Here's how the part is built. I have some questions about the finished solid (model axes, mm). A direction names the side the tool comes from. Coordinates: 2 decimals unless noted, no trailing zeros. Write each loop counter-clockwise with the first axis right and the second up, starting at its lowest first coordinate (ties: lowest second). Pieces come first, ordered by that corner, then holes. Notation, with made-up numbers: (27.5, 65) - (56.5, 65) arc R27 ccw to (56.5, 81) - close; hole circle Ø2 at (63, 72.25). An arc over 180 degrees is marked (long way). Answer in a Markdown table with one row per item. Add a question column.
Item 1: If I drill on probe 1 along Z at (x, y) = (-100, -157.5); probe 2 along Y at (x, z) = (-41.5, 47.5); probe 3 along Z at (x, y) = (31, -197.5), over which ranges is the centre line in solid material (lowest first)? Write a range as from..to.
Item 2: I'm going to push flat-ended pins straight in: pin 1 (20 mm diameter, centred on x = -41, z = 20.5, fed in from +Y); pin 2 (24.5 mm diameter, centred on x = -78, y = -129, fed in from -Z); pin 3 (12 mm diameter, centred on x = -72.5, z = -46.5, fed in from +Y). Where does each tip first touch, or does it pass through?
Item 3: We'd pull the mould along Z, two halves only. Please class faces 4 (the face through (-52, -140, -60)), 5 (the face through (-80, -141, 50)), 6 (the face through (-59.985, -83.479, 1.319)), 7 (the face through (-63, 3, -55)): +Z half, -Z half, draft (parallel to the pull), parting line (faces both ways), or undercut.
Item 4: Which directions (+Z, -Z, +X, -X, +Y, -Y) give clear straight access to the entire face, cutting with the end or side of a thin tool? Please do faces 1 (the face through (-61, -69, 0)), 2 (the face through (-83.3, -124.5, 55.1)), 3 (the face through (-68, -6, 50)).
Item 5: Imagine slicing it at C-C (z = 56). State how many separate pieces and enclosed holes the cut face has, plus the area to 3 significant figures.
Item 6: Imagine slicing it at A-A (x = -77). Please give me the cut outline in (y, z), plus the area to 3 significant figures.
Item 7: Imagine slicing it at B-B (y = -199.5). Please give me the cut outline in (x, z), plus the area to 3 significant figures.
from build123d import *

# Parameters (mm, degrees)
BOSS_EXTRUDE1_DEPTH      = 110
REVOLVE4_ANGLE           = 180
SKETCH5_R                = 2.5
BOSS_EXTRUDE2_DEPTH      = 120
CUT_EXTRUDE2_REACH       = 151.317
CUT_EXTRUDE2_END_RADIUS  = 50
REVOLVE5_ANGLE           = 180
CUT_EXTRUDE4_DEPTH       = 15
CUT_EXTRUDE5_DEPTH       = 85
CUT_EXTRUDE5_DEPTH_BACK  = 75
SKETCH7_5_W              = 21.213203436
SKETCH7_5_H              = 100
REVOLVE6_ANGLE           = 180
BOSS_EXTRUDE3_DEPTH      = 3
BOSS_EXTRUDE3_DEPTH_BACK = 10
SKETCH9_R                = 50
BOSS_EXTRUDE4_START      = -110
SKETCH9_3_R              = 50
BOSS_EXTRUDE4_DEPTH      = 13
BOSS_EXTRUDE5_DEPTH      = 120
CUT_EXTRUDE6_START       = -110
CUT_EXTRUDE6_DEPTH       = 20
CUT_EXTRUDE7_DEPTH       = 50
SKETCH9_5_R              = 7.5
BOSS_EXTRUDE6_DEPTH      = 10
BOSS_EXTRUDE7_START      = -110
SKETCH9_6_R              = 7.5
BOSS_EXTRUDE7_DEPTH      = 10
SKETCH12_R               = 12.571901436
CUT_EXTRUDE8_DEPTH       = 281.297435946
BOSS_EXTRUDE9_START      = 15
BOSS_EXTRUDE9_DEPTH      = 15


# Read off the part's stored shape, not the designer's step: Cut-Extrude6
with BuildPart() as part:
    # Sketch1 → Boss-Extrude1 (new body)
    with BuildSketch(Plane(origin=(0, 0, 0), x_dir=(1, 0, 0), z_dir=(0, 1, 0))):
        with BuildLine():
            Line((0, 60), (0, 50))
            ThreePointArc((0, 50), (-50, 0), (0, -50))
            Line((0, -50), (0, -60))
            ThreePointArc((0, -60), (-60, 0), (0, 60))
        make_face()
    extrude(amount=-BOSS_EXTRUDE1_DEPTH)

    # Sketch2 → Revolve4 (revolve)
    with BuildSketch(Plane(origin=(0, 0, 0), x_dir=(0, 0, -1), z_dir=(1, 0, 0))):
        with BuildLine():
            ThreePointArc((-7.741180955, 11.323216436), (-7.20664666, 11.680380834), (-7, 12.289142263))
            Line((-7, 12.289142263), (-7, 13.397459622))
            Line((-7, 13.397459622), (-5, 13.397459622))
            Line((-5, 13.397459622), (-5, 12.057713659))
            Line((-5, 12.057713659), (-5, 10.754488287))
            ThreePointArc((-5, 10.754488287), (-5.20664666, 10.145726858), (-5.741180955, 9.78856246))
            Line((-5.741180955, 9.78856246), (-49.872833452, -2.036478187))
            ThreePointArc((-49.872833452, -2.036478187), (-50.001126305, -2.061997222), (-50.131652498, -2.070552361))
            Line((-50.131652498, -2.070552361), (-60, -2.070552361))
            Line((-60, -2.070552361), (-60, 0))
            Line((-60, 0), (-50.131652498, 0))
            ThreePointArc((-50.131652498, 0), (-50.001126305, 0.008555139), (-49.872833452, 0.034074174))
            Line((-49.872833452, 0.034074174), (-7.741180955, 11.323216436))
        make_face()
    revolve(axis=Axis((0, 9.451262914, 0), (0, -1, 0)), revolution_arc=REVOLVE4_ANGLE)

    # Sketch5 → Boss-Extrude2 (add)
    with BuildSketch(Plane.XY.offset(60)):
        with BuildLine():
            Line((-60, -25), (0, -25))
            Line((0, -25), (0, -15))
            Line((0, -15), (0, 0))
            Line((0, 0), (-60, 0))
            Line((-60, 0), (-65.17766953, 5.17766953))
            ThreePointArc((-65.17766953, 5.17766953), (-68.713203436, 6.642135624), (-72.248737342, 5.17766953))
            Line((-72.248737342, 5.17766953), (-76.213203436, 1.213203436))
            Line((-76.213203436, 1.213203436), (-81.213203436, -3.786796564))
            Line((-81.213203436, -3.786796564), (-60, -25))
        make_face()
        with Locations((-68.713203436, 1.642135624)):
            Circle(SKETCH5_R, mode=Mode.SUBTRACT)
    extrude(amount=-BOSS_EXTRUDE2_DEPTH)

    # Cut-Extrude2: up to this cylinder (the profile starts inside it)
    cut_extrude2_end = Plane(origin=(0, -12.579447, 0), z_dir=(0, 1, 0)) * Cylinder(CUT_EXTRUDE2_END_RADIUS, 403.634, mode=Mode.PRIVATE)
    # Sketch6 → Cut-Extrude2 (cut, up to the surface)
    with BuildSketch(Plane(origin=(0, 0, 0), x_dir=(0, 0, -1), z_dir=(1, 0, 0)), mode=Mode.PRIVATE) as cut_extrude2_sk1:
        Polygon((-49.872833452, -2.036478187), (-50, -25), (50, -25), (49.872833452, -2.036478187), (42.27259339, 0), (-42.27259339, 0), align=None)
    cut_extrude2_tool1 = extrude(cut_extrude2_sk1.sketch, amount=-CUT_EXTRUDE2_REACH, mode=Mode.PRIVATE) & cut_extrude2_end
    add(cut_extrude2_tool1.solids().sort_by_distance((0, -12.579447, 0))[0], mode=Mode.SUBTRACT)

    # Sketch2<8> → Revolve5 (revolve)
    with BuildSketch(Plane(origin=(0, 0, 0), x_dir=(0, 0, -1), z_dir=(1, 0, 0))):
        with BuildLine():
            Line((-49.872833452, 0.034074174), (-7.741180955, 11.323216436))
            ThreePointArc((-7.741180955, 11.323216436), (-7.20664666, 11.680380834), (-7, 12.289142263))
            Line((-7, 12.289142263), (-7, 13.397459622))
            Line((-7, 13.397459622), (-5, 13.397459622))
            Line((-5, 13.397459622), (-5, 12.057713659))
            Line((-5, 12.057713659), (-5, 10.754488287))
            ThreePointArc((-5, 10.754488287), (-5.20664666, 10.145726858), (-5.741180955, 9.78856246))
            Line((-5.741180955, 9.78856246), (-49.872833452, -2.036478187))
            ThreePointArc((-49.872833452, -2.036478187), (-50.001126305, -2.061997222), (-50.131652498, -2.070552361))
            Line((-50.131652498, -2.070552361), (-60, -2.070552361))
            Line((-60, -2.070552361), (-60, 0))
            Line((-60, 0), (-50.131652498, 0))
            ThreePointArc((-50.131652498, 0), (-50.001126305, 0.008555139), (-49.872833452, 0.034074174))
        make_face()
    revolve(axis=Axis((0, 9.451262914, 0), (0, -1, 0)), revolution_arc=REVOLVE5_ANGLE)

    # Sketch7 → Cut-Extrude4 (cut)
    with BuildSketch(Plane(origin=(0, 0, 0), x_dir=(1, 0, 0), z_dir=(0, 1, 0))):
        with BuildLine():
            ThreePointArc((0, -50.131652498), (-50.131652498, 0), (0, 50.131652498))
            Line((0, 50.131652498), (0, 60))
            Line((0, 60), (-60, 60))
            Line((-60, 60), (-60, 50))
            Line((-60, 50), (-60, -50))
            Line((-60, -50), (-60, -60))
            Line((-60, -60), (0, -60))
            Line((0, -60), (0, -50.131652498))
        make_face()
    extrude(amount=-CUT_EXTRUDE4_DEPTH, mode=Mode.SUBTRACT)

    # Sketch7<5> → Cut-Extrude5 (cut, two sides: drawn at the far end of the back side and taken through both)
    with BuildSketch(Plane(origin=(0, 0, 0), x_dir=(1, 0, 0), z_dir=(0, 1, 0)).offset(-CUT_EXTRUDE5_DEPTH_BACK)):
        with Locations((-70.606601718, 0)):
            Rectangle(SKETCH7_5_W, SKETCH7_5_H)
    extrude(amount=CUT_EXTRUDE5_DEPTH + CUT_EXTRUDE5_DEPTH_BACK, mode=Mode.SUBTRACT)

    # Sketch8 → Revolve6 (revolve)
    with BuildSketch(Plane(origin=(0, 0, 0), x_dir=(0, 0, -1), z_dir=(1, 0, 0))):
        with BuildLine():
            Line((60, -77), (60, -82))
            Line((60, -82), (67.250339251, -82))
            ThreePointArc((67.250339251, -82), (69.750339251, -79.5), (67.250339251, -77))
            Line((67.250339251, -77), (60, -77))
        make_face()
        with BuildLine():
            Line((67.250339251, -85), (60, -85))
            Line((60, -85), (60, -90))
            Line((60, -90), (67.250339251, -90))
            ThreePointArc((67.250339251, -90), (69.750339251, -87.5), (67.250339251, -85))
        make_face()
        with BuildLine():
            Line((60, -69), (60, -74))
            Line((60, -74), (67.250339251, -74))
            ThreePointArc((67.250339251, -74), (69.750339251, -71.5), (67.250339251, -69))
            Line((67.250339251, -69), (60, -69))
        make_face()
    revolve(axis=Axis((0, -110, 0), (0, 1, 0)), revolution_arc=REVOLVE6_ANGLE)



with BuildPart() as body_2:
    # Sketch9 → Boss-Extrude3 (new, two sides: drawn at the far end of the back side and taken through both)
    with BuildSketch(Plane.XY.offset(60).offset(-BOSS_EXTRUDE3_DEPTH_BACK)):
        with Locations((0, -160)):
            Circle(SKETCH9_R)
    extrude(amount=BOSS_EXTRUDE3_DEPTH + BOSS_EXTRUDE3_DEPTH_BACK)


with BuildPart() as body_3:
    # Sketch9<3> → Boss-Extrude4 (new body)
    with BuildSketch(Plane.XY.offset(60).offset(BOSS_EXTRUDE4_START)):
        with Locations((0, -160)):
            Circle(SKETCH9_3_R)
    extrude(amount=-BOSS_EXTRUDE4_DEPTH)


with BuildPart() as part_1:
    add(part.part)

    add(body_2.part)  # Boss-Extrude5 merges body 2

    add(body_3.part)  # Boss-Extrude5 merges body 3
    # Sketch9<4> → Boss-Extrude5 (add)
    with BuildSketch(Plane.XY.offset(60)):
        with BuildLine():
            Line((-60, -111.049582772), (-60, -160))
            ThreePointArc((-60, -160), (-42.426406871, -202.426406871), (0, -220))
            Line((0, -220), (0, -210))
            ThreePointArc((0, -210), (-50, -160), (0, -110))
            Line((0, -110), (0, -90))
            Line((0, -90), (-60, -90))
            Line((-60, -90), (-60, -111.049582772))
        make_face()
    extrude(amount=-BOSS_EXTRUDE5_DEPTH)

    # Cut-Extrude6 outline → Cut-Extrude6 (cut)
    with BuildSketch(Plane(origin=(0, 0, 0), x_dir=(1, 0, 0), z_dir=(0, 1, 0)).offset(CUT_EXTRUDE6_START)):
        with BuildLine():
            Line((0, -50), (0, 50))
            ThreePointArc((0, 50), (-50, 0), (0, -50))
        make_face()
    extrude(amount=CUT_EXTRUDE6_DEPTH, mode=Mode.SUBTRACT)

    # Sketch11 → Cut-Extrude7 (cut)
    with BuildSketch(Plane(origin=(0, -110, 0), x_dir=(1, 0, 0), z_dir=(0, 1, 0))):
        with BuildLine():
            Line((0, -50), (0, 50))
            ThreePointArc((0, 50), (-50, 0), (0, -50))
        make_face()
    extrude(amount=-CUT_EXTRUDE7_DEPTH, mode=Mode.SUBTRACT)

    # Sketch9<5> → Boss-Extrude6 (add)
    with BuildSketch(Plane.XY.offset(60)):
        with BuildLine():
            ThreePointArc((-100, -160), (-111.591109915, -151.105828541), (-106, -137.607695155))
            Line((-106, -137.607695155), (-60, -111.049582772))
            Line((-60, -111.049582772), (-60, -160))
            Line((-60, -160), (-100, -160))
        make_face()
        with Locations((-100, -148)):
            Circle(SKETCH9_5_R, mode=Mode.SUBTRACT)
    extrude(amount=-BOSS_EXTRUDE6_DEPTH)

    # Sketch9<6> → Boss-Extrude7 (add)
    with BuildSketch(Plane.XY.offset(60).offset(BOSS_EXTRUDE7_START)):
        with BuildLine():
            ThreePointArc((-100, -160), (-111.591109915, -151.105828541), (-106, -137.607695155))
            Line((-106, -137.607695155), (-60, -111.049582772))
            Line((-60, -111.049582772), (-60, -160))
            Line((-60, -160), (-100, -160))
        make_face()
        with Locations((-100, -148)):
            Circle(SKETCH9_6_R, mode=Mode.SUBTRACT)
    extrude(amount=-BOSS_EXTRUDE7_DEPTH)

    # Sketch12 → Cut-Extrude8 (cut, through all)
    with BuildSketch(Plane.XY.offset(63)):
        with Locations((0, -160)):
            Circle(SKETCH12_R)
    extrude(amount=-CUT_EXTRUDE8_DEPTH, mode=Mode.SUBTRACT)

    # Sketch13 → Boss-Extrude9 (add)
    with BuildSketch(Plane(origin=(0, -15, 0), x_dir=(1, 0, 0), z_dir=(0, 1, 0)).offset(BOSS_EXTRUDE9_START)):
        with BuildLine():
            ThreePointArc((0, 60), (-60, 0), (0, -60))
            Line((0, -60), (0, -50.131652498))
            ThreePointArc((0, -50.131652498), (-50.131652498, 0), (0, 50.131652498))
            Line((0, 50.131652498), (0, 60))
        make_face()
    extrude(amount=-BOSS_EXTRUDE9_DEPTH)


solid = part_1.part
Here are the results:
| question | item | result |
|---|---|---|
| 1 | probe 1 | z = -60..-50, 50..60 |
| 1 | probe 2 | y = -203.33..-187.89, -132.11..-85, -82..-77, -74..-69, -25..-15 |
| 1 | probe 3 | z = -63..-50, 50..63 |
| 2 | pin 1 | stops at y = 3.79 |
| 2 | pin 2 | stops at z = -60 |
| 2 | pin 3 | stops at y = 6.64 |
| 3 | face 4 | -Z half |
| 3 | face 5 | undercut |
| 3 | face 6 | parting line |
| 3 | face 7 | draft |
| 4 | face 1 | -X |
| 4 | face 2 | +Z, -Z, -X |
| 4 | face 3 | -X, +Y, -Y |
| 5 | separate pieces | 1 |
| 5 | enclosed holes | 3 |
| 5 | area | 15,000 mm2 |
| 6 | outline | (-160, -60) - (-120.86, -60) - (-120.86, -50) - (-160, -50) - close; (-160, 50) - (-120.86, 50) - (-120.86, 60) - (-160, 60) - close; (-8, -60) - (0.43, -60) - (0.43, -50) - (-8, -50) - close; (-8, 50) - (0.43, 50) - (0.43, 60) - (-8, 60) - close |
| 6 | area | 951 mm2 |
| 7 | outline | (-45.16, -60) - (-30.66, -60) - (-30.66, -63) - (30.66, -63) - (30.66, -50) - (-30.66, -50) - (-30.66, 50) - (30.66, 50) - (30.66, 63) - (-30.66, 63) - (-30.66, 60) - (-45.16, 60) - close |
| 7 | area | 3,340 mm2 |
